Could you check a few things on this drawing? It's one solid part, dimensions in mm from its lowest x, y, z. Give positions to 0.01 mm unless a question says otherwise; leave off trailing zeros. Order: outer loops, then holes, each group sorted by start corner. A loop starts at its lowest first (then second) coordinate and runs counter-clockwise, first axis right, second up. Notation, with made-up numbers: (65, 68) -> (71, 68) arc R35 ccw to (71, 103) -> close; hole circle Ø3 at (13.25, 34.25). An arc over 180 degrees is marked (long way). Answer as a JSON object with one key per item and string values.
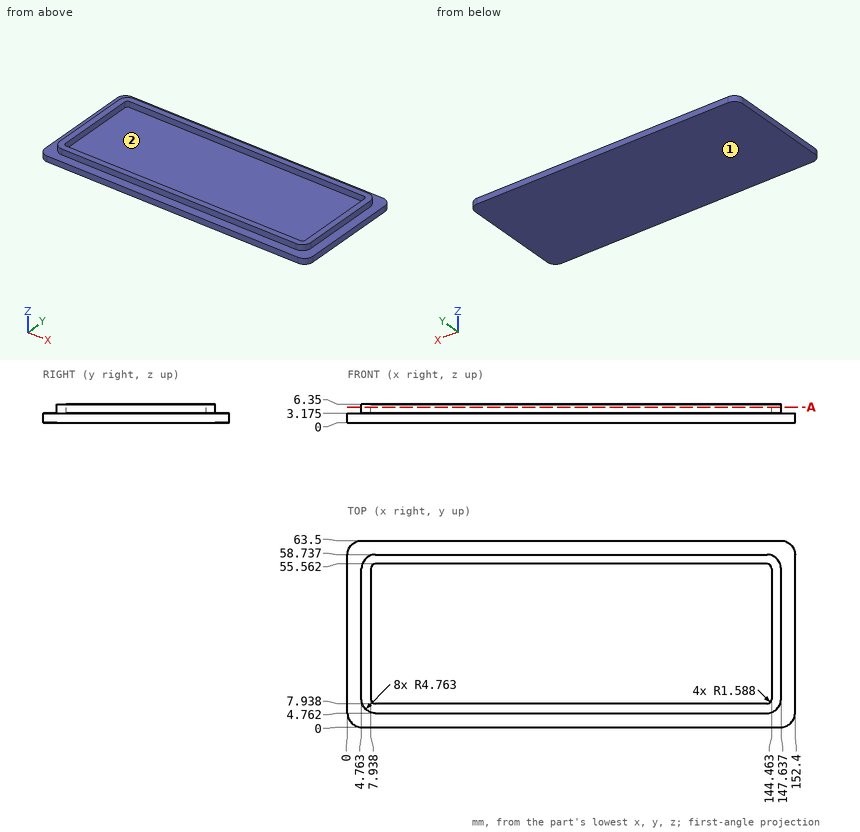
1. Please list where these lines run through material, in increasing order: L1, parallel to X at y = 34.5, z = 5.25; L2, parallel to Y at x = 113, z = 5.5; L3, parallel to Z at x = 9, y = 27 (1 decimal).
Worked answers:
{"L1": "4.76 to 7.94, 144.46 to 147.64", "L2": "4.76 to 7.94, 55.56 to 58.74", "L3": "0 to 3.2"}
2. If we mould it in two halves opening along Y, with no side actions, what happens to the marked faces 1 and 2? For each: +Y half, -Y half, draft (parallel to the pull), parting line (faces both ways), or undercut.
Worked answers:
{"face 1": "draft", "face 2": "undercut"}
3. If we section it at A-A on z = 5.25: Please give me the cut outline in (x, y) (1 decimal), then the cut area to 3 significant figures.
Worked answers:
{"outline": "(4.8, 9.5) arc R4.8 ccw to (9.5, 4.8) -> (142.9, 4.8) arc R4.8 ccw to (147.6, 9.5) -> (147.6, 54) arc R4.8 ccw to (142.9, 58.7) -> (9.5, 58.7) arc R4.8 ccw to (4.8, 54) -> close; hole (7.9, 9.5) arc R1.6 ccw to (9.5, 7.9) -> (142.9, 7.9) arc R1.6 ccw to (144.5, 9.5) -> (144.5, 54) arc R1.6 ccw to (142.9, 55.6) -> (9.5, 55.6) arc R1.6 ccw to (7.9, 54) -> close", "area": "1,190 mm²"}
4. Will these pins go through, and if not, where does the flat tip stop? pin 1 Ø1 at (y, z) = (28.5, 5.5) entering from -X; pin 2 Ø1 at (y, z) = (33.5, 4) entering from +X; pin 3 Ø4 at (x, y) = (43, 35) entering from +Z (1 decimal).
Worked answers:
{"pin 1": "x = 4.76", "pin 2": "x = 147.64", "pin 3": "z = 3.2"}
